For this review, take the finished solid that the model builds, in its own axes (mm). Round coordinates to 2 decimals unless told otherwise and drop trailing zeros. Order: outer loops, then holes, each group sorted by start corner. A loop starts at its lowest first (then second) coordinate and runs counter-clockwise, first axis right, second up. Notation, with made-up numbers: M 38.5,27.25 L 91.5,27.25 A29 ccw 91.5,54.25 Z; hole C 89,36.25 d3. An arc over 180 degrees is marked long. Use a Markdown table: item, result.
from build123d import *

# Parameters (mm, degrees)
SKETCH_1_W      = 180
SKETCH_1_H      = 98
SKETCH_1_R      = 6.2
SKETCH_1_R_2    = 8.2
SKETCH_1_R_3    = 1.5
SKETCH_1_R_4    = 1.6
SKETCH_1_R_5    = 3.6
SKETCH_1_W_2    = 12.2
SKETCH_1_H_2    = 12.2
SKETCH_1_W_3    = 46.5
SKETCH_1_H_3    = 36
EXTRUDE_1_DEPTH = 2.2
FILLET_1_R      = 1
FILLET_2_R      = 0.3


with BuildPart() as part:
    # Эскиз1 → Бобышка-Вытянуть1 (new body)
    with BuildSketch(Plane.XY):
        with Locations((49.911, 29.5)):
            Rectangle(SKETCH_1_W, SKETCH_1_H)
        with Locations((-24.089, 5.5)):
            Circle(SKETCH_1_R, mode=Mode.SUBTRACT)
        with Locations((123.911, 58.5)):
            Circle(SKETCH_1_R, mode=Mode.SUBTRACT)
        with Locations((123.911, 5.5)):
            Circle(SKETCH_1_R_2, mode=Mode.SUBTRACT)
        with Locations((-37.589, 76)):
            Circle(SKETCH_1_R_3, mode=Mode.SUBTRACT)
        with Locations((137.411, 76)):
            Circle(SKETCH_1_R_3, mode=Mode.SUBTRACT)
        with Locations((137.411, -17)):
            Circle(SKETCH_1_R_3, mode=Mode.SUBTRACT)
        with Locations((-37.589, -17)):
            Circle(SKETCH_1_R_3, mode=Mode.SUBTRACT)
        with Locations((3.556, 3.556)):
            Circle(SKETCH_1_R_4, mode=Mode.SUBTRACT)
        with Locations((3.556, 66.421)):
            Circle(SKETCH_1_R_4, mode=Mode.SUBTRACT)
        with Locations((96.266, 66.421)):
            Circle(SKETCH_1_R_4, mode=Mode.SUBTRACT)
        with Locations((96.266, 3.556)):
            Circle(SKETCH_1_R_4, mode=Mode.SUBTRACT)
        with Locations((8.255, 52.959)):
            Circle(SKETCH_1_R_5, mode=Mode.SUBTRACT)
        with Locations((91.567, 52.959)):
            Circle(SKETCH_1_R_5, mode=Mode.SUBTRACT)
        with Locations((-24.089, 30.5)):
            Circle(SKETCH_1_R_5, mode=Mode.SUBTRACT)
        with Locations((-24.089, -10.5)):
            Circle(SKETCH_1_R_5, mode=Mode.SUBTRACT)
        with Locations((38.7, 68)):
            Circle(SKETCH_1_R_3, mode=Mode.SUBTRACT)
        with Locations((16.891, 11.049)):
            Rectangle(SKETCH_1_W_2, SKETCH_1_H_2, mode=Mode.SUBTRACT)
        with Locations((38.1, 11.049)):
            Rectangle(SKETCH_1_W_2, SKETCH_1_H_2, mode=Mode.SUBTRACT)
        with Locations((61.722, 11.049)):
            Rectangle(SKETCH_1_W_2, SKETCH_1_H_2, mode=Mode.SUBTRACT)
        with Locations((82.931, 11.049)):
            Rectangle(SKETCH_1_W_2, SKETCH_1_H_2, mode=Mode.SUBTRACT)
        with Locations((49.75, 46)):
            Rectangle(SKETCH_1_W_3, SKETCH_1_H_3, mode=Mode.SUBTRACT)
        with BuildLine():
            Line((4.282953003, 36.1885), (12.282953003, 36.1885))
            ThreePointArc((12.282953003, 36.1885), (13.482953003, 34.9885), (12.282953003, 33.7885))
            Line((12.282953003, 33.7885), (4.282953003, 33.7885))
            ThreePointArc((4.282953003, 33.7885), (3.082953003, 34.9885), (4.282953003, 36.1885))
        make_face(mode=Mode.SUBTRACT)
        with BuildLine():
            Line((95.567, 33.7885), (87.567, 33.7885))
            ThreePointArc((87.567, 33.7885), (86.367, 34.9885), (87.567, 36.1885))
            Line((87.567, 36.1885), (95.567, 36.1885))
            ThreePointArc((95.567, 36.1885), (96.767, 34.9885), (95.567, 33.7885))
        make_face(mode=Mode.SUBTRACT)
        with BuildLine():
            Line((4.282953003, 32.1885), (12.282953003, 32.1885))
            ThreePointArc((12.282953003, 32.1885), (13.482953003, 30.9885), (12.282953003, 29.7885))
            Line((12.282953003, 29.7885), (4.282953003, 29.7885))
            ThreePointArc((4.282953003, 29.7885), (3.082953003, 30.9885), (4.282953003, 32.1885))
        make_face(mode=Mode.SUBTRACT)
        with BuildLine():
            Line((95.567, 29.7885), (87.567, 29.7885))
            ThreePointArc((87.567, 29.7885), (86.367, 30.9885), (87.567, 32.1885))
            Line((87.567, 32.1885), (95.567, 32.1885))
            ThreePointArc((95.567, 32.1885), (96.767, 30.9885), (95.567, 29.7885))
        make_face(mode=Mode.SUBTRACT)
        with BuildLine():
            Line((4.282953003, 28.1885), (12.282953003, 28.1885))
            ThreePointArc((12.282953003, 28.1885), (13.482953003, 26.9885), (12.282953003, 25.7885))
            Line((12.282953003, 25.7885), (4.282953003, 25.7885))
            ThreePointArc((4.282953003, 25.7885), (3.082953003, 26.9885), (4.282953003, 28.1885))
        make_face(mode=Mode.SUBTRACT)
        with BuildLine():
            Line((95.567, 25.7885), (87.567, 25.7885))
            ThreePointArc((87.567, 25.7885), (86.367, 26.9885), (87.567, 28.1885))
            Line((87.567, 28.1885), (95.567, 28.1885))
            ThreePointArc((95.567, 28.1885), (96.767, 26.9885), (95.567, 25.7885))
        make_face(mode=Mode.SUBTRACT)
        with BuildLine():
            Line((4.282953003, 24.1885), (12.282953003, 24.1885))
            ThreePointArc((12.282953003, 24.1885), (13.482953003, 22.9885), (12.282953003, 21.7885))
            Line((12.282953003, 21.7885), (4.282953003, 21.7885))
            ThreePointArc((4.282953003, 21.7885), (3.082953003, 22.9885), (4.282953003, 24.1885))
        make_face(mode=Mode.SUBTRACT)
        with BuildLine():
            Line((95.567, 21.7885), (87.567, 21.7885))
            ThreePointArc((87.567, 21.7885), (86.367, 22.9885), (87.567, 24.1885))
            Line((87.567, 24.1885), (95.567, 24.1885))
            ThreePointArc((95.567, 24.1885), (96.767, 22.9885), (95.567, 21.7885))
        make_face(mode=Mode.SUBTRACT)
    extrude(amount=EXTRUDE_1_DEPTH)

    # Скругление1
    fillet_1_edges = [part.edges().sort_by_distance(p)[0] for p in [
        (139.911, -19.5, 1.1),
        (-40.089, -19.5, 1.1),
        (-40.089, 78.5, 1.1),
        (139.911, 78.5, 1.1),
    ]]
    fillet(fillet_1_edges, radius=FILLET_1_R)

    # Скругление2
    fillet_2_edges = [part.edges().sort_by_distance(p)[0] for p in [
        (89.031, 4.949, 1.1),
        (89.031, 17.149, 1.1),
        (76.831, 17.149, 1.1),
        (76.831, 4.949, 1.1),
        (22.991, 4.949, 1.1),
        (22.991, 17.149, 1.1),
        (10.791, 17.149, 1.1),
        (10.791, 4.949, 1.1),
        (44.2, 4.949, 1.1),
        (44.2, 17.149, 1.1),
        (32, 17.149, 1.1),
        (32, 4.949, 1.1),
        (67.822, 4.949, 1.1),
        (67.822, 17.149, 1.1),
        (55.622, 17.149, 1.1),
        (55.622, 4.949, 1.1),
    ]]
    fillet(fillet_2_edges, radius=FILLET_2_R)


solid = part.part
Q1. Wall thickness on line 1 along X through (y, z) = (15, 0.95); line 2 along Y through (x, z) = (63.5, 1.8); line 3 along X through (y, z) = (23, 0.1): over which ranges is each line inside the solid? List them lowest first. Write a range as [from, to].
Determined:
| item | result |
|---|---|
| line 1 | x = [-40.09, 10.79], [22.99, 32], [44.2, 55.62], [67.82, 76.83], [89.03, 139.91] |
| line 2 | y = [-19.5, 4.95], [17.15, 28], [64, 78.5] |
| line 3 | x = [-40.09, 3.08], [13.48, 86.37], [96.77, 139.91] |
Q2. Draft analysis for pull direction Y (two halves, no side actions). For faces 1 (the flat face through (49, 19, 0)), 2 (the cylindrical face through (93.502, 55.995, 1.085)), state which applies: pulls with the +Y half, pulls with the -Y half, needs draft (parallel to the pull), parting line crosses it, or undercut.
Determined:
| item | result |
|---|---|
| face 1 | needs draft |
| face 2 | undercut |
Q3. Add section A-A (y = -10.5). Write out the cut boundary in (x, z), then the cut area to 3 significant figures.
Determined:
| item | result |
|---|---|
| outline | M -40.09,0 L -27.69,0 L -27.69,2.2 L -40.09,2.2 Z; M -20.49,0 L 139.91,0 L 139.91,2.2 L -20.49,2.2 Z |
| area | 380 mm^2 |
Q4. Clearance check with a flat-ended pin moving along its axis: pin 1 (6 mm diameter, centred on x = 8.255, y = 52.959, fed in from +Z). State where the tip first meets the part, or that it passes through.
Determined:
| item | result |
|---|---|
| pin 1 | passes through |
Q5. Add section B-B (z = 1.05). Give the number of separate pieces and of enclosed holes in the cut face, then the cut area to 3 significant figures.
Determined:
| item | result |
|---|---|
| separate pieces | 1 |
| enclosed holes | 29 |
| area | 14,500 mm^2 |
